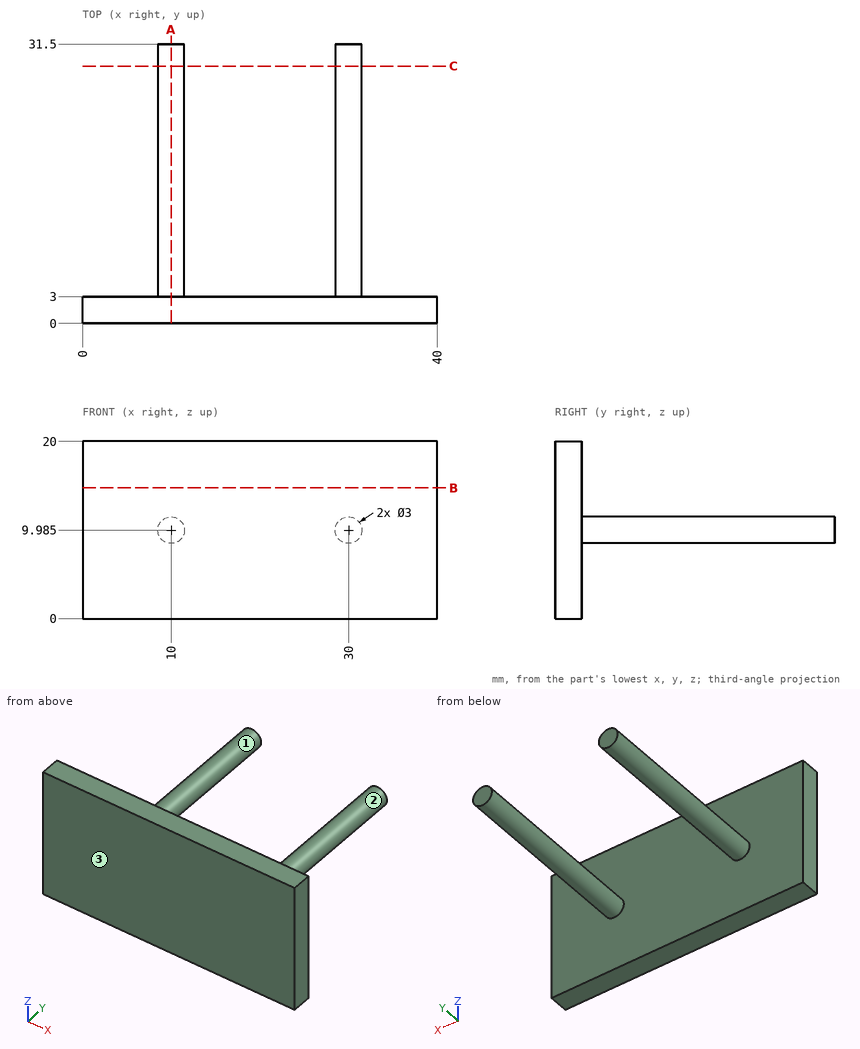
Job drawing, mm, ordinate dimensions from the low corner. One solid piece. Round coordinates to 2 decimals unless told otherwise and drop trailing zeros. Order: outer loops, then holes, each group sorted by start corner. A loop starts at its lowest first (then second) coordinate and runs counter-clockwise, first axis right, second up. Notation, with made-up numbers: (47.5, 80) -> (58.5, 80) arc R23 ccw to (58.5, 100) -> close; hole circle Ø2 at (75, 46). An arc over 180 degrees is marked (long way). Answer in a Markdown table with one row per item.
1) Pin check, flat tips, straight feed: P1, Ø1.5, axis at x = 6, y = 19, coming from the +Z side; P2, Ø4, axis at x = 9, y = 17, coming from the -Z side (1 decimal); P3, Ø4, axis at x = 28, y = 10, coming from the +Z side (1 decimal). Stop position of each tip, or through.
Values:
| item | result |
|---|---|
| P1 | through |
| P2 | z = 8.5 |
| P3 | z = 11.5 |
2) Mould opens along X. For the marked faces 1, 2 and 3 say: released by +X, released by -X, zero draft, split by the parting line, or undercut.
Values:
| item | result |
|---|---|
| face 1 | undercut |
| face 2 | undercut |
| face 3 | zero draft |
3) Band-saw the part on C-C on y = 29. Give the cut face in (x, z) (1 decimal).
Values:
| item | result |
|---|---|
| outline | circle Ø3 at (10, 10); circle Ø3 at (30, 10) |
4) Band-saw the part on B-B on z = 14.75. Give the cut face in (x, y), and give its area (3 significant figures).
Values:
| item | result |
|---|---|
| outline | (0, 0) -> (40, 0) -> (40, 3) -> (0, 3) -> close |
| area | 120 mm2 |
5) Wall check: L1, parallel to Y at x = 21.5, z = 16; L2, parallel to Z at x = 29.5, y = 29; L3, parallel to X at y = 15, z = 9. Give the ranges that are in metal, low to high.
Values:
| item | result |
|---|---|
| L1 | 0 to 3 |
| L2 | 8.57 to 11.4 |
| L3 | 8.87 to 11.13, 28.87 to 31.13 |
6) Band-saw the part on A-A on x = 10. Give the cut face in (y, z) (1 decimal).
Values:
| item | result |
|---|---|
| outline | (0, 0) -> (3, 0) -> (3, 8.5) -> (31.5, 8.5) -> (31.5, 11.5) -> (3, 11.5) -> (3, 20) -> (0, 20) -> close |
